Autodesk Fusion 360 part; units mm, degrees
sketch "Sketch1" plane through (0, 0, 0) normal (0, 0, 1) x (1, 0, 0)
  line L0 (33, -21) -> (-33, -21)
  line L1 (-33, -21) -> (-33, 21)
  line L2 (-33, 21) -> (33, 21)
  line L3 (33, 21) -> (33, -21)
  line L4 (33, -21) -> (-33, 21) construction
  line L5 (-33, -21) -> (33, 21) construction
  dimension "d1" = 66
  dimension "d2" = 42
extrude "Extrude1" add sketch "Sketch1" along normal blind 12
chamfer "Chamfer1" distance 12 angle 45 2 edges at (33, -21, 6) (33, 21, 6)
sketch "Sketch2" plane through (0, 0, 12) normal (0, 0, 1) x (-1, 0, 0)
  line L0 (-33, -9) -> (-21, -21)
  line L1 (-21, -21) -> (33, -21)
  line L2 (33, -21) -> (33, 21)
  line L3 (33, 21) -> (-21, 21)
  line L4 (-21, 21) -> (-33, 9)
  line L5 (-33, 9) -> (-33, -9)
  line L6 (33, -21) -> (21, -21)
  line L7 (21, -21) -> (21, 21)
  line L8 (21, 21) -> (33, 21)
  line L9 (33, 21) -> (33, -21)
  dimension "d6" = 12
extrude "Extrude2" add sketch "Sketch2" along normal blind 48 contours L1 L2 L3 L6 L7 L8 L9
fillet "Fillet1" radius 21 2 edges at (-27, 21, 60) (-27, -21, 60)
sketch "Sketch3" plane through (0, 0, 0) normal (0, 1, 0) x (1, 0, 0)
  line L0 (-21, -50) -> (-21, -12)
  line L1 (-21, -12) -> (33, -12)
  line L2 (33, -12) -> (-21, -50)
extrude "Extrude3" add sketch "Sketch3" along normal mid plane 12
equation "d7 = 60 mm - 12 mm"
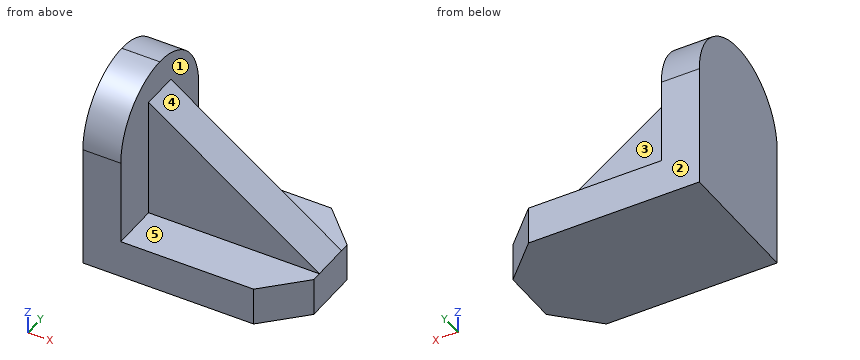
Design review of the part built by this model. Coordinates are the model's own, in mm. Face numbers are marked on the shaded views. A direction names the side the tool comes from. Coordinates: 2 decimals unless noted, no trailing zeros. Write each loop counter-clockwise with the first axis right and the second up, starting at its lowest first coordinate (ties: lowest second). Pieces come first, ordered by that corner, then holes. Notation, with made-up numbers: (-7.75, -1) -> (34.25, -1) arc R18 ccw to (34.25, 5) -> close; hole circle Ø8 at (78.5, 15). An arc over 180 degrees is marked (long way). Write each question's results on one line, items separated by ' | '. Start each with the question number.
(1) Take a section at A-A on x = 8.5. Write out the cut boundary in (y, z).
(2) Clearance check with flat-ended pins moving along their axes: P1, Ø10, axis at x = -12, z = 23, coming from the -Y side; P2, Ø19, axis at x = 12.5, z = 39.5, coming from the +Y side; P3, Ø16.5, axis at x = 12.5, y = -16, coming from the +Z side. State where each tip first meets the part, or that it passes through.
(3) For line 1 along Y through (x, z) = (-14, 37); line 2 along X through (y, z) = (15, 12.5); line 3 along Z through (x, y) = (30, 11), list the stretches that pass through material, from the lowest coordinate up. Write a range as from..to.
(4) Take a section at C-C on y = 10. Write out the cut boundary in (x, z), and give its area (3 significant figures).
(5) Take a section at D-D on y = -13. Write out the cut boundary in (x, z), and give its area (3 significant figures).
(6) Take a section at B-B on z = 18. Write out the cut boundary in (x, y), and give its area (3 significant figures).
(7) Tool access review of the marked faces 1, 2, 3, 4 and 5: name each direction out of +Z, -Z, +X, -X, +Y, -Y from which nothing blocks a thin tool from reaching the whole face with its end or side.
Results found:
1) outline: (-21, 0) -> (21, 0) -> (21, 12) -> (6, 12) -> (6, 29.24) -> (-6, 29.24) -> (-6, 12) -> (-21, 12) -> close
2) P1: stops at y = -6 | P2: passes through | P3: stops at z = 12
3) line 1: y = -6..6 | line 2: x = -33..-21 | line 3: z = 0..12
4) outline: (-33, 0) -> (32, 0) -> (32, 12) -> (-21, 12) -> (-21, 57.47) -> (-33, 57.47) -> close | area: 1,330 mm2
5) outline: (-33, 0) -> (29, 0) -> (29, 12) -> (-21, 12) -> (-21, 55.49) -> (-33, 55.49) -> close | area: 1,270 mm2
6) outline: (-33, -21) -> (-21, -21) -> (-21, -6) -> (24.47, -6) -> (24.47, 6) -> (-21, 6) -> (-21, 21) -> (-33, 21) -> close | area: 1,050 mm2
7) face 1: +Z, +X | face 2: +Z, -Z, +X, -X, +Y | face 3: +Z, +X, +Y | face 4: +Z, +X, +Y, -Y | face 5: +Z, +X, -Y
